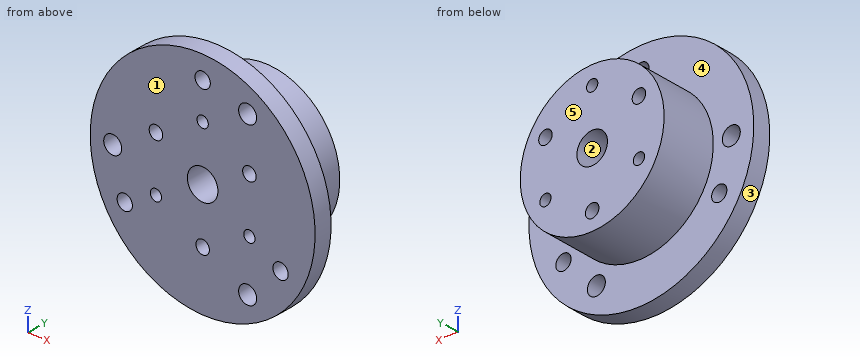
```python
from build123d import *

# Parameters (mm, degrees)
SKETCH1_R               = 25
BOSS_EXTRUDE1_DEPTH     = 4
F_4_0MM_DOWEL_HOLE1_D   = 4
M3_CLEARANCE_HOLE1_D    = 3.4
BOSS_EXTRUDE2_START     = -4
SKETCH9_R               = 16
BOSS_EXTRUDE2_DEPTH     = 16.3
TAP_DRILL_FOR_TAP1_D    = 6.8
F_3_0MM_DOWEL_HOLE1_D   = 3
TAP_DRILL_FOR_M3_TAP1_D = 2.5


with BuildPart() as part:
    # Sketch1 → Boss-Extrude1 (new body)
    with BuildSketch(Plane(origin=(0, 0, 0), x_dir=(1, 0, 0), z_dir=(0, 1, 0))):
        with Locations(Location((0, 0, 0), (0, 0, 270))):
            Circle(SKETCH1_R)
    extrude(amount=BOSS_EXTRUDE1_DEPTH)

    # Ø4.0mm Dowel Hole1 (through all)
    with Locations(Plane(origin=(0, 4, 0), x_dir=(1, 0, 0), z_dir=(0, 1, 0))):
        with Locations((10, -17.320508076), (-20, 0), (10, 17.320508076)):
            Hole(F_4_0MM_DOWEL_HOLE1_D / 2)

    # M3 Clearance Hole1 (through all)
    with Locations(Plane(origin=(0, 4, 0), x_dir=(1, 0, 0), z_dir=(0, 1, 0))):
        with Locations((17.320508076, 10), (0, -20), (-17.320508076, 10)):
            Hole(M3_CLEARANCE_HOLE1_D / 2)

    # Sketch9 → Boss-Extrude2 (add)
    with BuildSketch(Plane(origin=(0, 4, 0), x_dir=(1, 0, 0), z_dir=(0, 1, 0)).offset(BOSS_EXTRUDE2_START)):
        with Locations(Location((0, 0, 0), (0, 0, 270))):
            Circle(SKETCH9_R)
    extrude(amount=BOSS_EXTRUDE2_DEPTH)

    # Tap Drill for  Tap1 (through all)
    with Locations(Plane.XZ):
        with Locations((0, 0)):
            Hole(TAP_DRILL_FOR_TAP1_D / 2)

    # Ø3.0mm Dowel Hole1 (through all)
    with Locations(Plane(origin=(0, 16.3, 0), x_dir=(1, 0, 0), z_dir=(0, 1, 0))):
        with Locations((-10.392304845, -6), (0, 12), (10.392304845, -6)):
            Hole(F_3_0MM_DOWEL_HOLE1_D / 2)

    # Tap Drill for M3 Tap1 (through all)
    with Locations(Plane(origin=(0, 16.3, 0), x_dir=(1, 0, 0), z_dir=(0, 1, 0))):
        with Locations((10.392304845, 6), (0, -12), (-10.392304845, 6)):
            Hole(TAP_DRILL_FOR_M3_TAP1_D / 2)


solid = part.part
```
The listing builds one solid part. Answer for the finished solid, in the listing's coordinates (mm). Face numbers are marked on the shaded views. A direction names the side the tool comes from. Round coordinates to 2 decimals unless told otherwise and drop trailing zeros. Write each loop counter-clockwise with the first axis right and the second up, starting at its lowest first coordinate (ties: lowest second). Pieces come first, ordered by that corner, then holes. Notation, with made-up numbers: (23.5, -21.5) -> (59.5, -21.5) arc R25 cw to (59.5, 16.5) -> close; hole circle Ø2 at (-23.5, 27). An arc over 180 degrees is marked (long way). Write item = value, one per line.
1) Section D-D on z = 20 is taken. Write down the section's boundary in (x, y), plus the area to 3 significant figures.
Check values:
outline = (-15, 0) -> (-1.7, 0) -> (-1.7, 4) -> (-15, 4) -> close; (1.7, 0) -> (15, 0) -> (15, 4) -> (1.7, 4) -> close
area = 106 mm²
2) Section C-C on z = 0 is taken. Write down the section's boundary in (x, y), plus the area to 3 significant figures.
Check values:
outline = (-25, 0) -> (-22, 0) -> (-22, 4) -> (-25, 4) -> close; (-18, 0) -> (-3.4, 0) -> (-3.4, 16.3) -> (-16, 16.3) -> (-16, 4) -> (-18, 4) -> close; (3.4, 0) -> (25, 0) -> (25, 4) -> (16, 4) -> (16, 16.3) -> (3.4, 16.3) -> close
area = 467 mm²
3) Straight lines are drawn through the part: line 1 along Z through (x, y) = (10.5, 8.75); line 2 along Z through (x, y) = (10, 1.75); line 3 along X through (y, z) = (3.5, 5). For each, find the intervals that lie inside material, in ascending order. Write a range as [from, to].
Check values:
line_1 = [-12.07, -7.25], [-4.75, 4.5], [7.5, 12.07]
line_2 = [-22.91, -19.32], [-15.32, -7.19], [-4.81, 4.55], [7.45, 15.32], [19.32, 22.91]
line_3 = [-24.49, -11.51], [-9.27, 9.27], [11.51, 24.49]
4) Section A-A on x = -20 is taken. Write down the section's boundary in (y, z), plus the area to 3 significant figures.
Check values:
outline = (0, -15) -> (4, -15) -> (4, -2) -> (0, -2) -> close; (0, 2) -> (4, 2) -> (4, 15) -> (0, 15) -> close
area = 104 mm²
5) Which of the six approach directions +Z, -Z, +X, -X, +Y, -Y give full straight-line access (tool end or side, diameter ignored) to the marked faces 4 and 5?
Check values:
face_4 = +Y
face_5 = +Z, -Z, +X, -X, +Y
6) For a pull along X with two mould halves and no side action, classify the marked faces 1, 2 and 3 as released by +X, released by -X, zero draft, split by the parting line, or undercut.
Check values:
face_1 = zero draft
face_2 = undercut
face_3 = split by the parting line
7) Given pin 1 (1 mm diameter, centred on y = 13, z = -6.5, fed in from -X); pin 2 (2.5 mm diameter, centred on x = -10.39, z = 6, fed in from +Y); pin 3 (3 mm diameter, centred on y = 12.5, z = 2, fed in from -X); pin 4 (4 mm diameter, centred on y = 11.5, z = -5, fed in from -X), each flat-ended and moving along its own axis, determine where each tip first touches the part or whether it passes through.
Check values:
pin_1 = -14.83
pin_2 = through
pin_3 = -15.99
pin_4 = -15.72
8) Section B-B on y = 11.5 is taken. Write down the section's boundary in (x, z).
Check values:
outline = circle Ø32 at (0, 0); hole circle Ø3 at (-10.39, 6); hole circle Ø2.5 at (-10.39, -6); hole circle Ø6.8 at (0, 0); hole circle Ø3 at (0, -12); hole circle Ø2.5 at (0, 12); hole circle Ø3 at (10.39, 6); hole circle Ø2.5 at (10.39, -6)
